Could you check a few things on this drawing? It's one solid part, dimensions in mm from its lowest x, y, z. Give positions to 0.01 mm unless a question says otherwise; leave off trailing zeros. Order: outer loops, then holes, each group sorted by start corner. A loop starts at its lowest first (then second) coordinate and runs counter-clockwise, first axis right, second up.
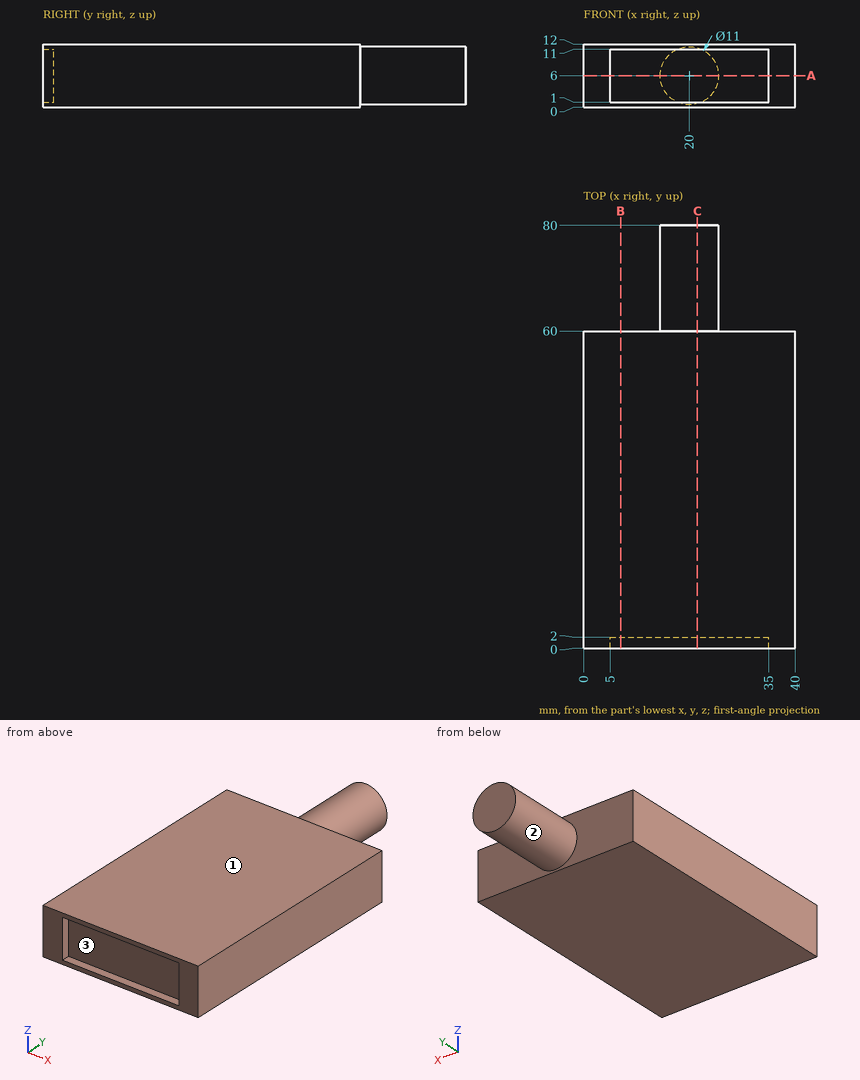
Q1. If we section it at C-C on x = 21.5: List the corners of the cut face in (y, z) for me.
Filled sheet:
outline: (0, 0) - (60, 0) - (60, 0.71) - (80, 0.71) - (80, 11.29) - (60, 11.29) - (60, 12) - (0, 12) - (0, 11) - (2, 11) - (2, 1) - (0, 1) - close
Q2. I need wall thicknesses on L1, parallel to Y at x = 23.5, z = 5.75; L2, parallel to Y at x = 2, z = 11.25; L3, parallel to X at y = 66, z = 1.25. Which ranges of each line are inside material? Lowest first, please.
Filled sheet:
L1: y = 2 to 80
L2: y = 0 to 60
L3: x = 17.23 to 22.77
Q3. If we section it at A-A on z = 6: List the corners of the cut face in (x, y) for me, plus the area to 3 significant figures.
Filled sheet:
outline: (0, 0) - (5, 0) - (5, 2) - (35, 2) - (35, 0) - (40, 0) - (40, 60) - (25.5, 60) - (25.5, 80) - (14.5, 80) - (14.5, 60) - (0, 60) - close
area: 2,560 mm2
Q4. I'm going to push flat-ended pins straight in: P1, Ø3.5, axis at x = 27.5, z = 6.5, coming from the +Y side; P2, Ø5, axis at x = 13.5, z = 7.5, coming from the -Y side. Where does each tip first touch, or does it pass through?
Filled sheet:
P1: stops at y = 60
P2: stops at y = 2
Q5. Thinking about a two-plate mould opening in X: for the marked faces 1, 2 and 3, which applies, released by +X, released by -X, zero draft, split by the parting line, or undercut?
Filled sheet:
face 1: zero draft
face 2: split by the parting line
face 3: undercut
Q6. If we section it at B-B on x = 7: List the corners of the cut face in (y, z) for me.
Filled sheet:
outline: (0, 0) - (60, 0) - (60, 12) - (0, 12) - (0, 11) - (2, 11) - (2, 1) - (0, 1) - close
